from build123d import *

# Parameters (mm, degrees)
F1_DEPTH  = 2
F3_DEPTH  = 3
F5_DEPTH  = 2
F7_DEPTH  = 3
F8_R      = 0.99999
F9_W      = 24
F9_H      = 22.6653645039
F10_DEPTH = 10
F11_W     = 24
F11_H     = 32
F11_W_2   = 8
F11_H_2   = 8
F12_DEPTH = 3
F13_R     = 1
F14_R     = 5
F15_W     = 24
F15_H     = 13.6653645039
F16_DEPTH = 2


# Not quite as in the source:
# - a fillet or chamfer is up to 0.001 mm smaller than in the source, because OpenCascade refuses the exact size


with BuildPart() as f1:
    # F0 (on Top) → F1 (new body)
    with BuildSketch(Plane.XY):
        with BuildLine():
            ThreePointArc((5.5, 1.5), (0, 24.1653645039), (-5.5, 1.5))
            Line((-5.5, 1.5), (-5.5, -1.5))
            ThreePointArc((-5.5, -1.5), (0, -24.1653645039), (5.5, -1.5))
            Line((5.5, -1.5), (5.5, 1.5))
        make_face()
    extrude(amount=F1_DEPTH)

    # F2 (on face) → F3 (join)
    with BuildSketch(Plane.XY.offset(2)):
        with BuildLine():
            Line((9.7844830762, 19.1125863177), (8.6602540378, 17.1653645039))
            ThreePointArc((8.6602540378, 17.1653645039), (9.4991255677, 9.0402063559), (4, 3.0002131139))
            Line((4, 3.0002131139), (4, -6.2432010007))
            Line((4, -6.2432010007), (9.1651513899, -16.1653645039))
            ThreePointArc((9.1651513899, -16.1653645039), (9.5868378212, -9.3206253964), (5.5, -3.8137179596))
            Line((5.5, -3.8137179596), (5.5, 1.5))
            ThreePointArc((5.5, 1.5), (11.6599594736, 9.3289327537), (9.7844830762, 19.1125863177))
        make_face()
        with BuildLine():
            ThreePointArc((-4, 3.0002131139), (-9.4991255677, 9.0402063559), (-8.6602540378, 17.1653645039))
            Line((-8.6602540378, 17.1653645039), (-9.7844830762, 19.1125863177))
            ThreePointArc((-9.7844830762, 19.1125863177), (-11.6599594736, 9.3289327537), (-5.5, 1.5))
            Line((-5.5, 1.5), (-5.5, -3.8137179596))
            ThreePointArc((-5.5, -3.8137179596), (-9.5868378212, -9.3206253964), (-9.1651513899, -16.1653645039))
            Line((-9.1651513899, -16.1653645039), (-4, -6.2432010007))
            Line((-4, -6.2432010007), (-4, 3.0002131139))
        make_face()
    extrude(amount=F3_DEPTH)

    # F4 (on face) → F5 (join)
    with BuildSketch(Plane.XY.offset(5)):
        with BuildLine():
            Line((-8.0717844057, 16.1461052023), (-9.7844830762, 19.1125863177))
            ThreePointArc((-9.7844830762, 19.1125863177), (-11.6599594736, 9.3289327537), (-5.5, 1.5))
            Line((-5.5, 1.5), (-5.5, -5.0414610795))
            ThreePointArc((-5.5, -5.0414610795), (-8.6043935433, -9.5263473097), (-8.5483759414, -14.980549891))
            Line((-8.5483759414, -14.980549891), (-4, -6.2432010007))
            Line((-4, -6.2432010007), (-4, 4.1031067556))
            ThreePointArc((-4, 4.1031067556), (-8.5258693153, 9.2827350759), (-8.0717844057, 16.1461052023))
        make_face()
        with BuildLine():
            ThreePointArc((5.5, 1.5), (11.6599594736, 9.3289327537), (9.7844830762, 19.1125863177))
            Line((9.7844830762, 19.1125863177), (8.0717844057, 16.1461052023))
            ThreePointArc((8.0717844057, 16.1461052023), (8.5258693153, 9.2827350759), (4, 4.1031067556))
            Line((4, 4.1031067556), (4, -6.2432010007))
            Line((4, -6.2432010007), (8.5483759414, -14.980549891))
            ThreePointArc((8.5483759414, -14.980549891), (8.6043935433, -9.5263473097), (5.5, -5.0414610795))
            Line((5.5, -5.0414610795), (5.5, 1.5))
        make_face()
    extrude(amount=F5_DEPTH)

    # F6 (on face) → F7 (join)
    with BuildSketch(Plane.XY.offset(7)):
        with BuildLine():
            Line((9.7844830762, 19.1125863177), (8.6602540378, 17.1653645039))
            ThreePointArc((8.6602540378, 17.1653645039), (9.4991255677, 9.0402063559), (4, 3.0002131139))
            Line((4, 3.0002131139), (4, -6.2432010007))
            Line((4, -6.2432010007), (9.1651513899, -16.1653645039))
            ThreePointArc((9.1651513899, -16.1653645039), (9.5868378212, -9.3206253964), (5.5, -3.8137179596))
            Line((5.5, -3.8137179596), (5.5, 1.5))
            ThreePointArc((5.5, 1.5), (11.6599594736, 9.3289327537), (9.7844830762, 19.1125863177))
        make_face()
        with BuildLine():
            ThreePointArc((-4, 3.0002131139), (-9.4991255677, 9.0402063559), (-8.6602540378, 17.1653645039))
            Line((-8.6602540378, 17.1653645039), (-9.7844830762, 19.1125863177))
            ThreePointArc((-9.7844830762, 19.1125863177), (-11.6599594736, 9.3289327537), (-5.5, 1.5))
            Line((-5.5, 1.5), (-5.5, -3.8137179596))
            ThreePointArc((-5.5, -3.8137179596), (-9.5868378212, -9.3206253964), (-9.1651513899, -16.1653645039))
            Line((-9.1651513899, -16.1653645039), (-4, -6.2432010007))
            Line((-4, -6.2432010007), (-4, 3.0002131139))
        make_face()
    extrude(amount=F7_DEPTH)

    # F8 (radius 1 in the source; OpenCascade refuses exactly that, so slightly less here)
    f8_edges = [f1.edges().sort_by_distance(p)[0] for p in [
        (8.525869, 9.282735, 7),
        (-8.525869, 9.282735, 7),
        (-8.525869, 9.282735, 5),
        (8.525869, 9.282735, 5),
        (-8.604394, -9.526347, 5),
        (-8.604394, -9.526347, 7),
        (8.604394, -9.526347, 7),
        (8.604394, -9.526347, 5),
    ]]
    fillet(f8_edges, radius=F8_R)

    # F9 (on face) → F10 (cut)
    with BuildSketch(Plane.XY.offset(10)):
        with Locations((0, -12.8326822519)):
            Rectangle(F9_W, F9_H)
    extrude(amount=-F10_DEPTH, mode=Mode.SUBTRACT)

    # F11 (on face) → F12 (join)
    with BuildSketch(Plane.XZ.offset(1.5)):
        with Locations((0, -4)):
            Rectangle(F11_W, F11_H)
        with Locations((0, 6)):
            Rectangle(F11_W_2, F11_H_2, mode=Mode.SUBTRACT)
    extrude(amount=F12_DEPTH)

    # F13
    f13_edges = [f1.edges().sort_by_distance(p)[0] for p in [
        (0, -4.5, 10),
        (4, -4.5, 6),
        (-4, -4.5, 6),
        (0, -4.5, 2),
    ]]
    fillet(f13_edges, radius=F13_R)

    # F14
    f14_edges = [f1.edges().sort_by_distance(p)[0] for p in [
        (-12, -3, 12),
        (12, -3, 12),
        (12, -3, -20),
        (-12, -3, -20),
    ]]
    fillet(f14_edges, radius=F14_R)

    # F15 (on face) → F16 (join)
    with BuildSketch(Plane(origin=(0, 0, 0), x_dir=(1, 0, 0), z_dir=(0, 0, -1))):
        with Locations((0, -5.3326822519)):
            Rectangle(F15_W, F15_H)
    extrude(amount=-F16_DEPTH)


solid = f1.part
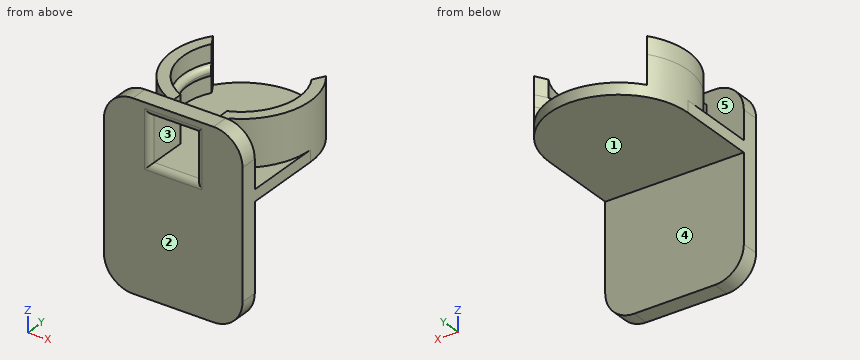
For this review, take the finished solid that the model builds, in its own axes (mm). Face numbers are marked on the shaded views. A direction names the side the tool comes from. Round coordinates to 2 decimals unless told otherwise and drop trailing zeros. Order: outer loops, then holes, each group sorted by start corner. A loop starts at its lowest first (then second) coordinate and runs counter-clockwise, first axis right, second up. Notation, with made-up numbers: M -30,-12 L -10,-12 A9 ccw -10,-7 Z; hole C 7.25,-22.5 d2. An arc over 180 degrees is marked long. Use a Markdown table: item, result. Add a question column.
Item 1: To check wall thickness, follow line 1 along Y through (x, z) = (1.25, -7); line 2 along Z through (x, y) = (5.5, 13.5); line 3 along X through (y, z) = (2, 6). State the ranges of each line that lie inside material, in increasing order.
Item 2: Insertion check: pin 1 (1.5 mm diameter, centred on x = 4.5, z = 2, fed in from +Y); pin 2 (8 mm diameter, centred on x = 6, y = 9.5, fed in from +Z); pin 3 (4 mm diameter, centred on x = 4, z = -11.5, fed in from +Y); pin 4 (8 mm diameter, centred on y = 10.5, z = -2.5, fed in from -X). Each pin has a flat end and moves straight along its axis. Give the tip position at first contact, or say it passes through.
Item 3: Mouldability with a two-part tool opening along Z and no side actions: class the marked faces 1, 2 and 3 as released by +Z, released by -Z, zero draft, split by the parting line, or undercut.
Item 4: Add section D-D, the plane z = -12.5. Give the boundary of the cut face in (x, y), then the cut area to 3 significant figures.
Item 5: Add section C-C, the plane z = 3.5. Give the boundary of the cut face in (x, y), then the cut area to 3 significant figures.
Item 6: Add section B-B, the plane z = 9.5. Give the boundary of the cut face in (x, y), then the cut area to 3 significant figures.
Item 7: Add section A-A, the plane x = 0. Give the boundary of the cut face in (y, z), then the cut area to 3 significant figures.
Item 8: Tool access review of the marked faces 4 and 5: name each direction out of +Z, -Z, +X, -X, +Y, -Y from which nothing blocks a thin tool from reaching the whole face with its end or side.
Geometry results:
| question | item | result |
|---|---|---|
| 1 | line 1 | y = -4.5 to -1.5 |
| 1 | line 2 | z = 0 to 2 |
| 1 | line 3 | x = -6.38 to -4, 4 to 6.38 |
| 2 | pin 1 | stops at y = 23.56 |
| 2 | pin 2 | stops at z = 10 |
| 2 | pin 3 | stops at y = -1.5 |
| 2 | pin 4 | stops at x = -12 |
| 3 | face 1 | released by -Z |
| 3 | face 2 | zero draft |
| 3 | face 3 | undercut |
| 4 | outline | M -12,-4.5 L 12,-4.5 L 12,-1.5 L -12,-1.5 Z |
| 4 | area | 72.0 mm² |
| 5 | outline | M -12,-4.5 L -5,-4.5 A1 ccw -4,-3.5 L -4,3 A10 cw -8.66,17.17 L -9.78,19.11 A12 ccw -5.5,1.5 L -5.5,-1.5 L -12,-1.5 Z; M 4,-3.5 A1 ccw 5,-4.5 L 12,-4.5 L 12,-1.5 L 5.5,-1.5 L 5.5,1.5 A12 ccw 9.78,19.11 L 8.66,17.17 A10 cw 4,3 Z |
| 5 | area | 134 mm² |
| 6 | outline | M -11.33,-4.5 L -5,-4.5 A1 ccw -4,-3.5 L -4,3 A10 cw -8.66,17.17 L -9.78,19.11 A12 ccw -5.5,1.5 L -5.5,-1.5 L -11.33,-1.5 Z; M 4,-3.5 A1 ccw 5,-4.5 L 11.33,-4.5 L 11.33,-1.5 L 5.5,-1.5 L 5.5,1.5 A12 ccw 9.78,19.11 L 8.66,17.17 A10 cw 4,3 Z |
| 6 | area | 130 mm² |
| 7 | outline | M -4.5,-20 L -1.5,-20 L -1.5,0 L 24.17,0 L 24.17,2 L -3.5,2 A1 ccw -4.5,1 Z; M -4.5,11 A1 ccw -3.5,10 L -1.5,10 L -1.5,12 L -4.5,12 Z |
| 7 | area | 123 mm² |
| 8 | face 4 | -Z, +X, -X, +Y |
| 8 | face 5 | +Z |
